```python
from build123d import *

# Parameters (mm, degrees)
HOLE_WIZARD_M4_1_D  = 3.3
CUT_EXTRUDE_1_DEPTH = 60.375921


with BuildPart() as part:
    # 草图1 → 旋转1 (revolve)
    with BuildSketch(Plane.XY, mode=Mode.PRIVATE) as revolve_1_sk:
        Polygon((-41.5, 0), (-39, 0), (-39, 5), (-32, 5), (-32, 9), (-40, 9), (-40, 1), (-41.5, 1), align=None)
    revolve(revolve_1_sk.sketch.rotate(Axis((0, 0, 0), (0, 1, 0)), 270), axis=Axis((0, 0, 0), (0, 1, 0)))

    # M4 螺纹孔1 (through all)
    with Locations(Plane(origin=(0, 9, 0), x_dir=(-1, 0, 0), z_dir=(0, 1, 0))):
        with Locations((0, -35.5), (30.743902, -17.75), (30.743902, 17.75), (0, 35.5), (-30.743902, 17.75), (-30.743902, -17.75)):
            Hole(HOLE_WIZARD_M4_1_D / 2)

    # 草图4 → 切除-拉伸1 (cut, through all)
    with BuildSketch(Plane(origin=(0, 9, 0), x_dir=(1, 0, 0), z_dir=(0, 1, 0))):
        with BuildLine():
            ThreePointArc((-32.451037, 14.694564), (-27.712813, 16), (-28.951384, 20.75614))
            ThreePointArc((-28.951384, 20.75614), (-30.374691, 22.843063), (-29.699519, 25.277235))
            ThreePointArc((-29.699519, 25.277235), (-19.5, 33.774991), (-7.040968, 38.359155))
            ThreePointArc((-7.040968, 38.359155), (0, 39), (7.040968, 38.359155))
            ThreePointArc((7.040968, 38.359155), (19.5, 33.774991), (29.699519, 25.277235))
            ThreePointArc((29.699519, 25.277235), (30.374691, 22.843063), (28.951384, 20.75614))
            ThreePointArc((28.951384, 20.75614), (27.712813, 16), (32.451037, 14.694564))
            ThreePointArc((32.451037, 14.694564), (34.970019, 14.883723), (36.740487, 13.08192))
            ThreePointArc((36.740487, 13.08192), (39, 0), (36.740487, -13.08192))
            ThreePointArc((36.740487, -13.08192), (34.970019, -14.883723), (32.451037, -14.694564))
            ThreePointArc((32.451037, -14.694564), (27.712813, -16), (28.951384, -20.75614))
            ThreePointArc((28.951384, -20.75614), (30.374691, -22.843063), (29.699519, -25.277235))
            ThreePointArc((29.699519, -25.277235), (19.5, -33.774991), (7.040968, -38.359155))
            ThreePointArc((7.040968, -38.359155), (0, -39), (-7.040968, -38.359155))
            ThreePointArc((-7.040968, -38.359155), (-19.5, -33.774991), (-29.699519, -25.277235))
            ThreePointArc((-29.699519, -25.277235), (-30.374691, -22.843063), (-28.951384, -20.75614))
            ThreePointArc((-28.951384, -20.75614), (-27.712813, -16), (-32.451037, -14.694564))
            ThreePointArc((-32.451037, -14.694564), (-34.970019, -14.883723), (-36.740487, -13.08192))
            ThreePointArc((-36.740487, -13.08192), (-39, 0), (-36.740487, 13.08192))
            ThreePointArc((-36.740487, 13.08192), (-34.970019, 14.883723), (-32.451037, 14.694564))
        make_face()
    extrude(amount=-CUT_EXTRUDE_1_DEPTH, mode=Mode.SUBTRACT)


solid = part.part
```
Verification items for the finished model (mm, model axes). A direction names the side the tool comes from. Round coordinates to 2 decimals unless told otherwise and drop trailing zeros. Order: outer loops, then holes, each group sorted by start corner. A loop starts at its lowest first (then second) coordinate and runs counter-clockwise, first axis right, second up. Notation, with made-up numbers: (52, -36.75) - (68, -36.75) arc R16 ccw to (68, -16.75) - close; hole circle Ø7 at (82, 65.5). An arc over 180 degrees is marked (long way). Use CSV: the item, a comma, the result in double quotes.
(1) Mould release check, pull along X, two halves, no side actions. Record for faces 4 (the face through (31, 0, -24)), 5 (the face through (-35.004, 7.028, -14.871)), 6 (the face through (-27.752, 7.028, -15.934)), 7 (the face through (-12.465, 0.493, -39.584)): released by +X, released by -X, zero draft, split by the parting line, or undercut.
Entries:
face 4,"zero draft"
face 5,"undercut"
face 6,"undercut"
face 7,"split by the parting line"
(2) Section check A-A on z = 0. Record the boundary of the cut face in (x, y), and give its area (3 significant figures).
Entries:
outline,"(-41.5, 0) - (-39, 0) - (-39, 9) - (-40, 9) - (-40, 1) - (-41.5, 1) - close; (39, 0) - (41.5, 0) - (41.5, 1) - (40, 1) - (40, 9) - (39, 9) - close"
area,"21.0 mm^2"
(3) Section check B-B on x = 0. Record the boundary of the cut face in (y, z).
Entries:
outline,"(0, -41.5) - (1, -41.5) - (1, -40) - (9, -40) - (9, -39) - (0, -39) - close; (0, 39) - (9, 39) - (9, 40) - (1, 40) - (1, 41.5) - (0, 41.5) - close"
(4) Thickness scan on probe 1 along X at (y, z) = (7, 18); probe 2 along Z at (x, y) = (29.5, 8.75); probe 3 along Z at (x, y) = (-29, 5.25). Record the ranges inside material, lowest first. Write a range as from..to.
Entries:
probe 1,"-35.72..-32.37, -29.11..-27.25, 27.25..29.11, 32.37..35.72"
probe 2,"-27.01..-25.51, -21.18..-18.83, -16.67..-14.48, 14.48..16.67, 18.83..21.18, 25.51..27.01"
probe 3,"-27.55..-26.08, -20.79..-14.72, 14.72..20.79, 26.08..27.55"
(5) Gauge pin test, flat ends, axial feed: pin 1 Ø3 at (x, z) = (30.74, 17.75) entering from -Y; pin 2 Ø4 at (x, z) = (-30.74, -17.75) entering from -Y; pin 3 Ø4 at (x, y) = (-23, 3.5) entering from -Z. Record the tip position at first contact, or that the pin passes through.
Entries:
pin 1,"through"
pin 2,"y = 5"
pin 3,"z = -34.04"
(6) Access from +Z, -Z, +X, -X, +Y, -Y to the whole of each face (thin tool, end or side, straight path). Record for faces 1 (the face through (39.05, 4.94, 8.67)), 2 (the face through (31.9, 5, 19.3)), 3 (the face through (-30.37, 6.56, -22.81)).
Entries:
face 1,"+Y"
face 2,"-Y"
face 3,"+Y, -Y"
(7) Section check D-D on y = 6.5. Record the boundary of the cut face in (x, z).
Entries:
outline,"circle Ø80 at (0, 0); hole (-36.74, -13.08) arc R3 ccw to (-32.45, -14.69) arc R3.5 cw to (-28.95, -20.76) arc R3 ccw to (-29.7, -25.28) arc R39 ccw to (-7.04, -38.36) arc R39 ccw to (7.04, -38.36) arc R39 ccw to (29.7, -25.28) arc R3 ccw to (28.95, -20.76) arc R3.5 cw to (32.45, -14.69) arc R3 ccw to (36.74, -13.08) arc R39 ccw to (36.74, 13.08) arc R3 ccw to (32.45, 14.69) arc R3.5 cw to (28.95, 20.76) arc R3 ccw to (29.7, 25.28) arc R39 ccw to (7.04, 38.36) arc R39 ccw to (-7.04, 38.36) arc R39 ccw to (-29.7, 25.28) arc R3 ccw to (-28.95, 20.76) arc R3.5 cw to (-32.45, 14.69) arc R3 ccw to (-36.74, 13.08) arc R39 ccw to start; hole circle Ø3.3 at (-30.74, -17.75); hole circle Ø3.3 at (-30.74, 17.75); hole circle Ø3.3 at (30.74, -17.75); hole circle Ø3.3 at (30.74, 17.75)"
